Autodesk Inventor part; units mm, degrees
ref_plane "РабПлоскость5" through (0, -2.5, 0) normal (0, 1, 0) x (-1, 0, 0)
ref_plane "YZ Plane" through (0, 0, 0) normal (1, 0, 0) x (0, 1, 0)
ref_plane "XZ Plane" through (0, 0, 0) normal (0, 1, 0) x (-1, 0, 0)
sketch "Эскиз1" plane through (0, 0, 0) normal (0, 1, 0) x (-1, 0, 0)
  line L0 (-23, 30) -> (23, 30)
  line L1 (23, 30) -> (23, -30)
  line L2 (23, -30) -> (-23, -30)
  line L3 (-23, -30) -> (-23, 30)
  line L4 (-18, 30) -> (18, 30)
  line L5 (18, 30) -> (18, -30)
  line L6 (18, -30) -> (-18, -30)
  line L7 (-18, -30) -> (-18, 30)
  point P0 (0, 0)
  point P1 (-18, 30)
  point P2 (-18, -30)
  dimension "d0" = 46
  dimension "d2" = 36
  dimension "d3" = 60
  dimension "d14" = 5
extrude "Выдавливание3" add sketch "Эскиз1" against normal blind 5 contours L0 L5 L2 L7
extrude "Выдавливание4" add sketch "Эскиз1" against normal blind 75 contours L0 L7 L2 L3 | L0 L1 L2 L5
ref_plane "РабПлоскость5" through (0, -2.5, 0) normal (0, 1, 0) x (-1, 0, 0)
sketch "Эскиз3" plane through (0, -75, 0) normal (0, -1, 0) x (1, 0, 0)
  line L0 (-18, 30) -> (-23, 30)
  line L1 (-23, -30) -> (-18, -30)
  point P0 (0, 0)
  point P1 (-20.322, 15)
  point P2 (-20.4927, -15)
  point P3 (20.6897, -15.1643)
  dimension "d59" = 15
  dimension "d60" = 15
sketch "Эскиз4" plane through (0, -75, 0) normal (0, -1, 0) x (1, 0, 0)
  line L0 (-23, -30) -> (-18, -30)
  line L1 (-18, -30) -> (-18, 30)
  point P0 (0, 0)
  point P1 (-20.5, -15)
  dimension "d43" = 15
  dimension "d44" = 2.5
hole "Отверстие3" at (-20.5, -75, -15) direction (0, 1, 0) diameter 2.459 depth 8.8 tip angle 118
hole "Отверстие4" at (-20.322, -75, 15) direction (0, 1, 0) diameter 2.459 depth 8.8 tip angle 118
sketch "Эскиз5" plane through (0, -75, 0) normal (0, -1, 0) x (1, 0, 0)
  circle A0 centre (-20.322, 15) radius 1.2295 construction
  circle A1 centre (-20.5, -15) radius 1.2295
  point P0 (0, 0)
  point P1 (20.4588, 15)
  point P2 (20.4588, -15)
hole "Отверстие5" at (20.4588, -75, 15) at (20.4588, -75, -15) direction (0, 1, 0) diameter 2.459 depth 8.8 tip angle 118
sketch "Эскиз9" plane through (23, 0, -30) normal (0, 0, -1) x (-1, 0, 0)
  point P0 (23, 0)
  point P1 (23.0428, -2.5128)
hole "Отверстие7" at (-0.0428, -2.5128, -30) direction (0, 0, 1) diameter 2.459 depth 8.8 tip angle 118
sketch "Эскиз8" plane through (23, 0, -30) normal (0, 0, -1) x (-1, 0, 0)
  line L0 (0, 0) -> (0, -75)
  line L1 (0, 0) -> (46, 0) construction
  line L2 (46, 0) -> (46, -75)
  line L3 (5, -5) -> (5, -75)
  line L4 (3.7707, -75) -> (1.3117, -75)
  line L5 (2.5, -75) -> (2.5, 0) construction
  line L6 (46, 0) -> (46, -75) construction
  line L7 (46, -2.5) -> (0, -2.5) construction
  line L8 (44.7295, -75) -> (42.2705, -75) construction
  line L9 (43.5, -75) -> (43.5, 0) construction
  line L10 (2.5, -20) -> (43.5, -20) construction
  line L11 (43.5, -20) -> (43.5, -55) construction
  line L12 (43.5, -55) -> (2.5, -55) construction
  line L13 (2.5, -55) -> (2.5, -20) construction
  line L14 (0, -75) -> (0, 0)
  line L15 (0, 0) -> (46, 0)
  line L16 (46, 0) -> (46, -75)
  line L17 (46, -75) -> (41, -75)
  line L18 (41, -75) -> (41, -5)
  line L19 (41, -5) -> (5, -5)
  line L20 (5, -5) -> (5, -75)
  line L21 (5, -75) -> (0, -75)
  circle A0 centre (23.0428, -2.5128) radius 1.2295
  point P0 (23, 0)
  dimension "d76" = 5
  dimension "d84" = 35
hole "Отверстие9" at (20.5, -55, -30) direction (0, 0, 1) diameter 2.459 depth 8.8 tip angle 118
hole "Отверстие10" at (-20.5, -55, -30) at (20.5, -20, -30) direction (0, 0, 1) diameter 2.459 depth 8.8 tip angle 118
hole "Отверстие11" at (-20.5, -20, -30) direction (0, 0, 1) diameter 2.459 depth 8.8 tip angle 118
chamfer "Фаска1" distance 2 angle 45 2 edges at (23, 0, 0) (-23, 0, 0)
equation "\"Радиус_гибки\" = Толщина"
equation "\"Ширина_просечки\" = Толщина"
equation "\"Глубина_просечки\" = 0.5 * Толщина"
equation "\"Радиус_перехода\" = Радиус_гибки"
equation "\"Радиус_Якоби\" = Радиус_гибки"
equation "\"Размер_зазора\" = Толщина"
properties part number "magnetGuide" material "Железо, мягкое"
The model under review builds one solid part; all positions refer to its coordinate system, in mm. A direction names the side the tool comes from. Round coordinates to 2 decimals unless told otherwise and drop trailing zeros. Order: outer loops, then holes, each group sorted by start corner. A loop starts at its lowest first (then second) coordinate and runs counter-clockwise, first axis right, second up.
(1) Take a section at C-C, the plane x = -7. State the section outline as (y, z) points.
Working result:
outline: (-5, -30) - (0, -30) - (0, 30) - (-5, 30) - close
(2) Mouldability with a two-part tool opening along X and no side actions: class faces 1 (the face through (21, -75, 0)), 2 (the face through (-0.41, -1.34, -25.54)), 3 (the face through (-23, -38, 0)) as released by +X, released by -X, zero draft, split by the parting line, or undercut.
Working result:
face 1: zero draft
face 2: undercut
face 3: released by -X
(3) Tool access review of faces 4 (the face through (0, -5, 0)), 5 (the face through (22, -1, 0)), 6 (the face through (20.93, -70.538, 13.864)): name each direction out of +Z, -Z, +X, -X, +Y, -Y from which nothing blocks a thin tool from reaching the whole face with its end or side.
Working result:
face 4: +Z, -Z, -Y
face 5: +Z, -Z, +X, +Y
face 6: -Y
(4) For P1, Ø8, axis at x = 8, z = -23.5, coming from the -Y side; P2, Ø2, axis at x = -20.5, y = -20, coming from the -Z side, all flat-tipped, find the tip position at first contact; note any pin that passes through.
Working result:
P1: stops at y = -5
P2: stops at z = -21.06
(5) Wall thickness on L1, parallel to X at y = -71, z = -15; L2, parallel to X at y = -20, z = -22.75; L3, parallel to X at y = -63.5, z = 23.5: over which ranges is each line inside the solid? List them lowest first.
Working result:
L1: x = -23 to -21.73, -19.27 to -18, 18 to 19.23, 21.69 to 23
L2: x = -23 to -21.73, -19.27 to -18, 18 to 19.27, 21.73 to 23
L3: x = -23 to -18, 18 to 23
(6) Take a section at B-B, the plane z = 26.5. State the section outline as (x, y) points.
Working result:
outline: (-23, -75) - (-18, -75) - (-18, -5) - (18, -5) - (18, -75) - (23, -75) - (23, -2) - (21, 0) - (-21, 0) - (-23, -2) - close
(7) Take a section at A-A, the plane y = -36. State the section outline as (x, z) points.
Working result:
outline: (-23, -30) - (-18, -30) - (-18, 30) - (-23, 30) - close; (18, -30) - (23, -30) - (23, 30) - (18, 30) - close
